from build123d import *

# Parameters (mm, degrees)
SKETCH1_W           = 40
SKETCH1_H           = 20
BOSS_EXTRUDE1_DEPTH = 20
SKETCH2_R           = 2.75
CUT_EXTRUDE1_DEPTH  = 21
SKETCH3_R           = 5
CUT_EXTRUDE2_DEPTH  = 5
SKETCH4_R           = 4
CUT_EXTRUDE3_DEPTH  = 5.5
SKETCH5_R           = 4
CUT_EXTRUDE4_DEPTH  = 5.5
SKETCH6_R           = 3.5
CUT_EXTRUDE5_DEPTH  = 15.5


with BuildPart() as part:
    # Sketch1 → Boss-Extrude1 (new body)
    with BuildSketch(Plane.XY):
        with Locations((20, 10)):
            Rectangle(SKETCH1_W, SKETCH1_H)
    extrude(amount=BOSS_EXTRUDE1_DEPTH)

    # Sketch2 → Cut-Extrude1 (cut, through all)
    with BuildSketch(Plane(origin=(0, 20, 0), x_dir=(1, 0, 0), z_dir=(0, 1, 0))):
        with Locations((8, -10)):
            Circle(SKETCH2_R)
        with Locations((32, -10)):
            Circle(SKETCH2_R)
    extrude(amount=-CUT_EXTRUDE1_DEPTH, mode=Mode.SUBTRACT)

    # Sketch3 → Cut-Extrude2 (cut)
    with BuildSketch(Plane(origin=(0, 20, 0), x_dir=(1, 0, 0), z_dir=(0, 1, 0))):
        with Locations((8, -10)):
            Circle(SKETCH3_R)
        with Locations((32, -10)):
            Circle(SKETCH3_R)
    extrude(amount=-CUT_EXTRUDE2_DEPTH, mode=Mode.SUBTRACT)

    # Sketch4 → Cut-Extrude3 (cut)
    with BuildSketch(Plane.XY.offset(20)):
        with Locations((20, 10)):
            Circle(SKETCH4_R)
    extrude(amount=-CUT_EXTRUDE3_DEPTH, mode=Mode.SUBTRACT)

    # Sketch5 → Cut-Extrude4 (cut)
    with BuildSketch(Plane(origin=(0, 0, 0), x_dir=(-1, 0, 0), z_dir=(0, 0, -1))):
        with Locations((-20, 10)):
            Circle(SKETCH5_R)
    extrude(amount=-CUT_EXTRUDE4_DEPTH, mode=Mode.SUBTRACT)

    # Sketch6 → Cut-Extrude5 (cut, through all)
    with BuildSketch(Plane.XY.offset(14.5)):
        with Locations((20, 10)):
            Circle(SKETCH6_R)
    extrude(amount=-CUT_EXTRUDE5_DEPTH, mode=Mode.SUBTRACT)


solid = part.part
Could you check a few things on this model? Use its own coordinates, in mm. A direction names the side the tool comes from. Coordinates: 2 decimals unless noted, no trailing zeros. Order: outer loops, then holes, each group sorted by start corner. A loop starts at its lowest first (then second) coordinate and runs counter-clockwise, first axis right, second up.
Q1. Suppose I cut it at D-D on z = 17.25. Please give me the cut outline in (x, y).
Q2. Please list where these lines run through material, in increasing order: L1, parallel to X at y = 16.6, z = 10; L2, parallel to Z at x = 32, y = 9.75; L3, parallel to X at y = 17.25, z = 7.
Q3. Suppose I cut it at C-C on x = 20. Please give me the cut outline in (y, z).
Q4. Will these pins go through, and if not, where does the flat tip stop? pin 1 (3 mm diameter, centred on x = 6.5, z = 9.5, fed in from +Y); pin 2 (4.5 mm diameter, centred on x = 8, z = 10, fed in from -Y).
Q5. Suppose I cut it at B-B on z = 10. Please give me the cut outline in (x, y), and give its area (3 significant figures).
Q6. Thinking about a two-plate mould opening in Y: for faces 1 (the flat face through (20, 0, 10)), 2 (the flat face through (40, 10, 10)), 3 (the cylindrical face through (24, 10, 3)), which applies, released by +Y, released by -Y, zero draft, split by the parting line, or undercut?
Q7. Suppose I cut it at A-A on y = 10. Please give me the cut outline in (x, z).
Q8. Which directions (+Z, -Z, +X, -X, +Y, -Y) give clear straight access to the entire face, cutting with the end or side of a thin tool? Please do faces 4 (the cylindrical face through (21.615, 6.895, 10.063)), 5 (the cylindrical face through (19.479, 13.966, 17.288)), 6 (the cylindrical face through (27, 18, 10)).
Answer:
1. outline: (0, 0) - (40, 0) - (40, 20) - (0, 20) - close; hole circle Ø8 at (20, 10)
2. L1: x = 0 to 3, 13 to 27, 37 to 40
2. L2: z = 0 to 7.25, 12.75 to 20
2. L3: x = 0 to 4, 12 to 28, 36 to 40
3. outline: (0, 0) - (6, 0) - (6, 5.5) - (6.5, 5.5) - (6.5, 14.5) - (6, 14.5) - (6, 20) - (0, 20) - close; (13.5, 5.5) - (14, 5.5) - (14, 0) - (20, 0) - (20, 20) - (14, 20) - (14, 14.5) - (13.5, 14.5) - close
4. pin 1: stops at y = 15
4. pin 2: passes through
5. outline: (0, 0) - (5.25, 0) - (5.25, 15) - (3, 15) - (3, 20) - (0, 20) - close; (10.75, 0) - (29.25, 0) - (29.25, 15) - (27, 15) - (27, 20) - (13, 20) - (13, 15) - (10.75, 15) - close; (34.75, 0) - (40, 0) - (40, 20) - (37, 20) - (37, 15) - (34.75, 15) - close; hole circle Ø7 at (20, 10)
5. area: 497 mm2
6. face 1: released by -Y
6. face 2: zero draft
6. face 3: undercut
7. outline: (0, 0) - (16, 0) - (16, 5.5) - (16.5, 5.5) - (16.5, 14.5) - (16, 14.5) - (16, 20) - (0, 20) - close; (23.5, 5.5) - (24, 5.5) - (24, 0) - (40, 0) - (40, 20) - (24, 20) - (24, 14.5) - (23.5, 14.5) - close; hole circle Ø5.5 at (8, 10); hole circle Ø5.5 at (32, 10)
8. face 4: +Z, -Z
8. face 5: +Z
8. face 6: +Y
